Could you check a few things on this model? Use its own coordinates, in mm. A direction names the side the tool comes from. Coordinates: 2 decimals unless noted, no trailing zeros. Loops run counter-clockwise (first coordinate to the right, second up) from the corner with the lowest first, then second, coordinate; pieces in that order, holes last.
from build123d import *

# Parameters (mm, degrees)
F1_DEPTH = 5.4
F3_DEPTH = 4.4
F4_DEPTH = 0.7


with BuildPart() as f1:
    # F0 (on Top) → F1 (new body)
    with BuildSketch(Plane.XY):
        with BuildLine():
            Line((-13, -6.5), (-9.0593873965, -6.5))
            ThreePointArc((-9.0593873965, -6.5), (-8.4928156006, -7.2245818685), (-7.8684496567, -7.9))
            Line((-7.8684496567, -7.9), (7.8684496567, -7.9))
            ThreePointArc((7.8684496567, -7.9), (11.15, 0), (7.8684496567, 7.9))
            Line((7.8684496567, 7.9), (-7.8684496567, 7.9))
            ThreePointArc((-7.8684496567, 7.9), (-8.4928156006, 7.2245818685), (-9.0593873965, 6.5))
            Line((-9.0593873965, 6.5), (-13, 6.5))
            Line((-13, 6.5), (-13, 3.8))
            Line((-13, 3.8), (-12.5, 3.8))
            Line((-12.5, 3.8), (-12.5, -3.8))
            Line((-12.5, -3.8), (-13, -3.8))
            Line((-13, -3.8), (-13, -6.5))
        make_face()
    extrude(amount=F1_DEPTH)

    # F2 (on face) → F3 (cut)
    with BuildSketch(Plane.XY.offset(5.4)):
        with BuildLine():
            ThreePointArc((6.3727937359, -7.9), (9.1571381015, -4.3782784049), (10.15, 0))
            ThreePointArc((10.15, 0), (9.1571381015, 4.3782784049), (6.3727937359, 7.9))
            Line((6.3727937359, 7.9), (-6.3727937359, 7.9))
            ThreePointArc((-6.3727937359, 7.9), (-10.15, 0), (-6.3727937359, -7.9))
            Line((-6.3727937359, -7.9), (6.3727937359, -7.9))
        make_face()
    extrude(amount=-F3_DEPTH, mode=Mode.SUBTRACT)

    # F4 (cut): a face of the model
    f4_faces = [f1.faces().sort_by_distance(p)[0] for p in [
        (-10.7326109912, 0, 5.4),
    ]]
    extrude(f4_faces, amount=-F4_DEPTH, mode=Mode.SUBTRACT)


solid = f1.part
(1) Which directions (+Z, -Z, +X, -X, +Y, -Y) give clear straight access to the entire face, cutting with the end or side of a thin tool? Please do faces 1 (the face through (-8.484, 7.234, 2.317)), 2 (the face through (-11, -6.5, 2)), 3 (the face through (-10.5, 0.1, 4.7)), 4 (the face through (-12.5, 0, 2)).
Answers:
face 1: +Z, -Z, -X, +Y
face 2: +Z, -Z, -X, -Y
face 3: +Z, -X, +Y, -Y
face 4: +Z, -Z, -X
(2) I need wall thicknesses on probe 1 along Z at (x, y) = (-11, 1.75); probe 2 along Z at (x, y) = (1, 2.25); probe 3 along X at (y, z) = (4, 2.7). Which ranges of each line are inside material? Lowest first, please.
Answers:
probe 1: z = 0 to 4.7
probe 2: z = 0 to 1
probe 3: x = -13 to -9.33, 9.33 to 10.41
(3) Imagine slicing it at C-C, the plane y = -2.75. Write out the boundary of the cut face in (x, z), and give its area (3 significant figures).
Answers:
outline: (-12.5, 0) - (10.81, 0) - (10.81, 5.4) - (9.77, 5.4) - (9.77, 1) - (-9.77, 1) - (-9.77, 4.7) - (-12.5, 4.7) - close
area: 38.0 mm2
(4) Imagine slicing it at A-A, the plane z = 1.55. Write out the boundary of the cut face in (x, y), and give its area (3 significant figures).
Answers:
outline: (-13, -6.5) - (-9.06, -6.5) arc R11.15 ccw to (-7.87, -7.9) - (-6.37, -7.9) arc R10.15 cw to (-6.37, 7.9) - (-7.87, 7.9) arc R11.15 ccw to (-9.06, 6.5) - (-13, 6.5) - (-13, 3.8) - (-12.5, 3.8) - (-12.5, -3.8) - (-13, -3.8) - close; (6.37, -7.9) - (7.87, -7.9) arc R11.15 ccw to (7.87, 7.9) - (6.37, 7.9) arc R10.15 cw to start
area: 64.6 mm2
(5) For pin 1 (3 mm diameter, centred on x = -10.5, z = 3, fed in from +Y); pin 2 (4.5 mm diameter, centred on x = -3, y = 3.5, fed in from +Z); pin 3 (3 mm diameter, centred on x = -11, z = 2.5, fed in from -Y); pin 4 (1 mm diameter, centred on x = -5, z = 3, fed in from +Y), each with a flat end and sliding along its axis, tell me the tip position at first contact or that it passes through.
Answers:
pin 1: stops at y = 6.58
pin 2: stops at z = 1
pin 3: stops at y = -6.5
pin 4: passes through
(6) Imagine slicing it at B-B, the plane z = 0.45. Write out the boundary of the cut face in (x, y).
Answers:
outline: (-13, -6.5) - (-9.06, -6.5) arc R11.15 ccw to (-7.87, -7.9) - (7.87, -7.9) arc R11.15 ccw to (7.87, 7.9) - (-7.87, 7.9) arc R11.15 ccw to (-9.06, 6.5) - (-13, 6.5) - (-13, 3.8) - (-12.5, 3.8) - (-12.5, -3.8) - (-13, -3.8) - close
(7) We'd pull the mould along Y, two halves only. Please class faces 5 (the face through (0, 0, 1)), 6 (the face through (-11, 6.5, 2)), 7 (the face through (-13, -5, 2)), 8 (the face through (-10.15, 0.13, 2.88)): +Y half, -Y half, draft (parallel to the pull), parting line (faces both ways), or undercut.
Answers:
face 5: undercut
face 6: +Y half
face 7: draft
face 8: undercut
(8) Imagine slicing it at D-D, the plane x = 9. Write out the boundary of the cut face in (y, z), and give its area (3 significant figures).
Answers:
outline: (-6.58, 0) - (6.58, 0) - (6.58, 5.4) - (4.69, 5.4) - (4.69, 1) - (-4.69, 1) - (-4.69, 5.4) - (-6.58, 5.4) - close
area: 29.8 mm2
